```python
from build123d import *

# Parameters (mm, degrees)
SKETCH2_W               = 21
SKETCH2_H               = 21
SKETCH2_R               = 8
BOSS_EXTRUDE1_DEPTH     = 0.5
CUT_EXTRUDE1_START      = -1.5
CUT_EXTRUDE1_DEPTH      = 1.5
SKETCH4_W               = 21
SKETCH4_H               = 9
BOSS_EXTRUDE2_DEPTH     = 0.5
CUT_EXTRUDE2_DEPTH      = 26.563646062
CUT_EXTRUDE2_DEPTH_BACK = 26.563646062
SKETCH5_W               = 5
SKETCH5_H               = 5
CUT_EXTRUDE3_DEPTH      = 1.5
FILLET1_R               = 1
FILLET2_R               = 0.5
EXTRUDE_THIN1_DEPTH     = 4.5
FILLET3_R               = 0.5
FILLET4_R               = 1
CUT_EXTRUDE4_DEPTH      = 27.807046038
CUT_EXTRUDE4_DEPTH_BACK = 27.807046038
SKETCH8_W               = 5
SKETCH8_H               = 5
FILLET5_R               = 0.5
FILLET6_R               = 1


with BuildPart() as part:
    # Sketch2 → Boss-Extrude1 (new body)
    with BuildSketch(Plane(origin=(0, 0, 0), x_dir=(1, 0, 0), z_dir=(0, 1, 0))):
        Rectangle(SKETCH2_W, SKETCH2_H)
        with Locations(Location((0, 0, 0), (0, 0, 270))):
            Circle(SKETCH2_R, mode=Mode.SUBTRACT)
    extrude(amount=BOSS_EXTRUDE1_DEPTH)

    # Sketch3 → Cut-Extrude1 (cut)
    with BuildSketch(Plane(origin=(0, 0.5, 0), x_dir=(1, 0, 0), z_dir=(0, 1, 0)).offset(CUT_EXTRUDE1_START)):
        with BuildLine():
            Line((-8, 0), (-8, 10.5))
            Line((-8, 10.5), (-8, 11.595978523))
            Line((-8, 11.595978523), (8, 11.595978523))
            Line((8, 11.595978523), (8, 0))
            ThreePointArc((8, 0), (0, -8), (-8, 0))
        make_face()
    extrude(amount=CUT_EXTRUDE1_DEPTH, mode=Mode.SUBTRACT)

    # Sketch4 → Boss-Extrude2 (add)
    with BuildSketch(Plane(origin=(10.5, 0, 0), x_dir=(0, 0, -1), z_dir=(1, 0, 0))):
        with Locations((0, 4.5)):
            Rectangle(SKETCH4_W, SKETCH4_H)
    boss_extrude2 = extrude(amount=BOSS_EXTRUDE2_DEPTH)

    # Sketch5 → Cut-Extrude2 (cut, two sides: drawn at the far end of the back side and taken through both)
    with BuildSketch(Plane(origin=(11, 0, 0), x_dir=(0, 0, -1), z_dir=(1, 0, 0)).offset(-CUT_EXTRUDE2_DEPTH_BACK)):
        with Locations((0, 6.5)):
            Rectangle(SKETCH5_W, SKETCH5_H)
    extrude(amount=CUT_EXTRUDE2_DEPTH + CUT_EXTRUDE2_DEPTH_BACK, mode=Mode.SUBTRACT)

    # Sketch6 → Cut-Extrude3 (cut)
    with BuildSketch(Plane(origin=(11, 0, 0), x_dir=(0, 0, -1), z_dir=(1, 0, 0))):
        Polygon((10.5, 5), (4.5, 9), (4.5, 12.483472669), (11.734785125, 12.483472669), (11.734785125, 5), align=None)
    cut_extrude3 = extrude(amount=-CUT_EXTRUDE3_DEPTH, mode=Mode.SUBTRACT)

    # Mirror1: Cut-Extrude3 across plane
    add(cut_extrude3.mirror(Plane.XY), mode=Mode.SUBTRACT)

    # Fillet1
    fillet1_edges = [part.edges().sort_by_distance(p)[0] for p in [
        (11, 0, 0),
    ]]
    fillet(fillet1_edges, radius=FILLET1_R)

    # Fillet2
    fillet2_edges = [part.edges().sort_by_distance(p)[0] for p in [
        (10.5, 0.5, 0),
    ]]
    fillet(fillet2_edges, radius=FILLET2_R)

    # Sketch7 → Extrude-Thin1 (add, symmetric)
    with BuildSketch(Plane.XY):
        Polygon((11, 9), (11, 9.896446609), (11.633883476, 10.530330086), (11.280330086, 10.883883476), (10.5, 10.103553391), (10.5, 9), align=None)
    extrude_thin1 = extrude(amount=EXTRUDE_THIN1_DEPTH, both=True)

    # Fillet3
    fillet3_edges = [part.edges().sort_by_distance(p)[0] for p in [
        (11, 9.896446609, 0),
    ]]
    fillet(fillet3_edges, radius=FILLET3_R)

    # Fillet4
    fillet4_edges = [part.edges().sort_by_distance(p)[0] for p in [
        (10.5, 10.103553391, 0),
    ]]
    fillet(fillet4_edges, radius=FILLET4_R)

    # Mirror2: Boss-Extrude2, Extrude-Thin1 across plane
    add(boss_extrude2.mirror(Plane(origin=(0, 0, 0), x_dir=(0, 0, 1), z_dir=(1, 0, 0))))
    add(extrude_thin1.mirror(Plane(origin=(0, 0, 0), x_dir=(0, 0, 1), z_dir=(1, 0, 0))))

    # Sketch8 → Cut-Extrude4 (cut, two sides: drawn at the far end of the back side and taken through both)
    with BuildSketch(Plane(origin=(-10.5, 0, 0), x_dir=(0, 0, -1), z_dir=(1, 0, 0)).offset(-CUT_EXTRUDE4_DEPTH_BACK)):
        Polygon((4.5, 9), (4.5, 13.510449082), (11.904854474, 13.510449082), (11.904854474, 4.985722932), (10.5, 5), align=None)
        with Locations((0, 6.5)):
            Rectangle(SKETCH8_W, SKETCH8_H)
        Polygon((-10.5, 5), (-4.5, 9), (-4.5, 13.510449082), (-11.904854474, 13.510449082), (-11.904854474, 4.985722932), align=None)
    extrude(amount=CUT_EXTRUDE4_DEPTH + CUT_EXTRUDE4_DEPTH_BACK, mode=Mode.SUBTRACT)

    # Fillet5
    fillet5_edges = [part.edges().sort_by_distance(p)[0] for p in [
        (-10.5, 0.5, 0),
        (-11, 9.896446609, 0),
    ]]
    fillet(fillet5_edges, radius=FILLET5_R)

    # Fillet6
    fillet6_edges = [part.edges().sort_by_distance(p)[0] for p in [
        (-11, 0, 0),
        (-10.5, 10.103553391, 0),
    ]]
    fillet(fillet6_edges, radius=FILLET6_R)


solid = part.part
```
Geometry: final body of the model. Coordinates: model frame, mm. A direction names the side the tool comes from. Give positions to 0.01 mm unless a question says otherwise; leave off trailing zeros. Loops run counter-clockwise (first coordinate to the right, second up) from the corner with the lowest first, then second, coordinate; pieces in that order, holes last. Notation, with made-up numbers: (38, 61) -> (57, 61) arc R17 cw to (57, 89) -> close; hole circle Ø11 at (24, 23). An arc over 180 degrees is marked (long way). Use one line per item in the form item = value.
Item 1: Draft query along X for faces 1 (the face through (-11, 3, 0)), 2 (the face through (10.5, 3, 0)), 3 (the face through (10.9, 10, -4.5)). Return one class per face: pulls with the +X half, pulls with the -X half, needs draft (parallel to the pull), parting line crosses it, or undercut.
A:
face_1 = pulls with the -X half
face_2 = undercut
face_3 = needs draft
Item 2: Section query A-A on y = 3.5. Output: boundary loops of the cut face in (x, z), and give its area (3 significant figures).
A:
outline = (-11, -10.5) -> (-10.5, -10.5) -> (-10.5, 10.5) -> (-11, 10.5) -> close; (10.5, -10.5) -> (11, -10.5) -> (11, 10.5) -> (10.5, 10.5) -> close
area = 21.0 mm^2
Item 3: Section query D-D on z = -3. Output: boundary loops of the cut face in (x, y).
A:
outline = (-11.63, 10.53) -> (-11.15, 10.04) arc R0.5 cw to (-11, 9.69) -> (-11, 1) arc R1 ccw to (-10, 0) -> (-8, 0) -> (-8, 0.5) -> (-10, 0.5) arc R0.5 cw to (-10.5, 1) -> (-10.5, 9.69) arc R1 ccw to (-10.79, 10.4) -> (-11.28, 10.88) -> close; (8, 0) -> (10, 0) arc R1 ccw to (11, 1) -> (11, 9.69) arc R0.5 cw to (11.15, 10.04) -> (11.63, 10.53) -> (11.28, 10.88) -> (10.79, 10.4) arc R1 ccw to (10.5, 9.69) -> (10.5, 1) arc R0.5 cw to (10, 0.5) -> (8, 0.5) -> close
Item 4: Section query B-B on z = -0.5. Give the number of separate pieces and of enclosed holes in the cut face, and give its area (3 significant figures).
A:
separate_pieces = 4
enclosed_holes = 0
area = 8.15 mm^2
Item 5: Pin query (flat end, axial travel): P1, Ø3, axis at y = 2.5, z = 8, coming from the +X side; P2, Ø1.2, axis at x = -11, y = 9.5, coming from the -Z side; P3, Ø5, axis at y = 6.5, z = 5, coming from the -X side. Return the tip coordinate at first contact, or that it passes through.
A:
P1 = 11
P2 = -4.65
P3 = -11
Item 6: Line query: probe 1 along X at (y, z) = (2.5, 2.25); probe 2 along Y at (x, z) = (9.75, -5.25); probe 3 along X at (y, z) = (0.75, -5.5). Output: solid intervals per line, ascending.
A:
probe_1 = -11 to -10.5, 10.5 to 11
probe_2 = 0 to 0.5
probe_3 = -10.97 to -10.43, 10.43 to 10.97
Item 7: Access query for faces 4 (the face through (-10.9, 10, 4.5)), 5 (the face through (-10.9, 10, -4.5)), 6 (the face through (-10.5, 3, 0)), 7 (the face through (11, 3, 0)). Directions: +Z, -Z, +X, -X, +Y, -Y. A direction counts if a zero-diameter tool reaches every point of the face in a straight line with its end or side. Return the directions, or none.
A:
face_4 = +Z, +X, -X, +Y
face_5 = -Z, +X, -X, +Y
face_6 = +Z, -Z, +Y
face_7 = +Z, -Z, +X, -Y
Item 8: Section query C-C on y = 8. Output: boundary loops of the cut face in (x, z), and give its area (3 significant figures).
A:
outline = (-11, -6) -> (-10.5, -6) -> (-10.5, -2.5) -> (-11, -2.5) -> close; (-11, 2.5) -> (-10.5, 2.5) -> (-10.5, 6) -> (-11, 6) -> close; (10.5, -6) -> (11, -6) -> (11, -2.5) -> (10.5, -2.5) -> close; (10.5, 2.5) -> (11, 2.5) -> (11, 6) -> (10.5, 6) -> close
area = 7.00 mm^2
